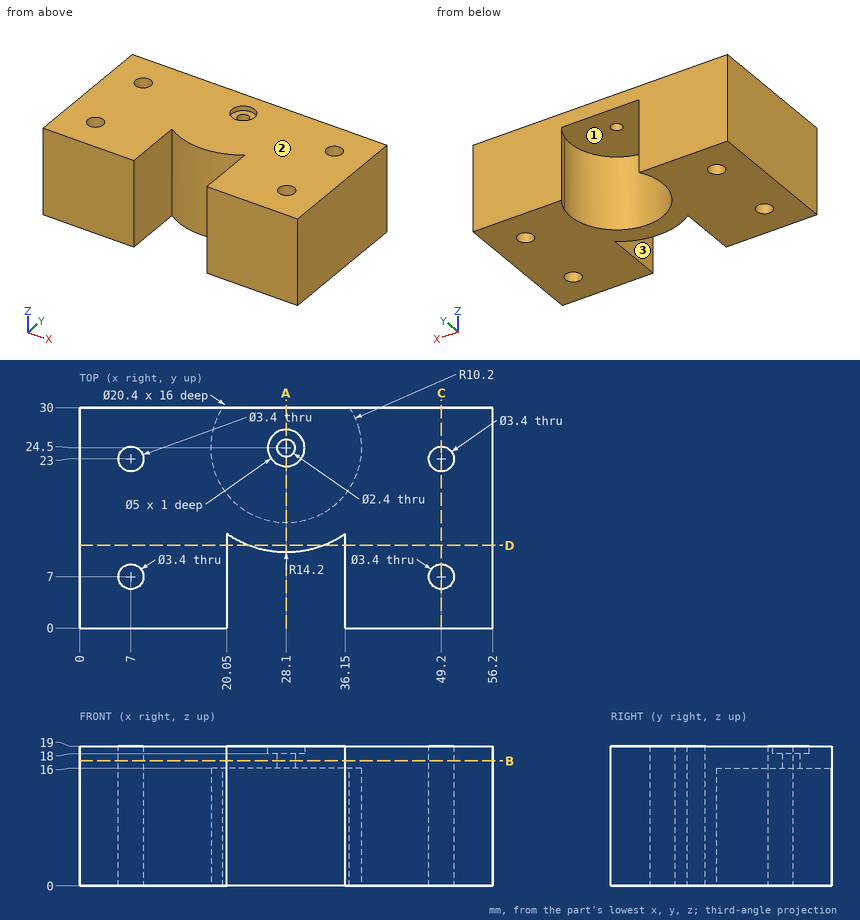
Print and shaded views of the part. All mm, measured from the part's lowest x, y and z. A direction names the side the tool comes from. Coordinates: 2 decimals unless noted, no trailing zeros. Write each loop counter-clockwise with the first axis right and the second up, starting at its lowest first coordinate (ties: lowest second). Pieces come first, ordered by that corner, then holes.
(1) Cut at B-B, the plane z = 17. List the corners of the cut face in (x, y), and give its area (3 significant figures).
(2) Flat gauge pins, fed straight in: pin 1 (5 mm diameter, centred on x = 33.5, z = 5.5, fed in from +Y); pin 2 (3 mm diameter, centred on x = 23, z = 9.5, fed in from +Y); pin 3 (12 mm diameter, centred on x = 28.1, y = 24.5, fed in from -Z). Where does each tip first touch, or does it go through?
(3) Drill centre lines: probe 1 along Y at (x, z) = (49.2, 7); probe 2 along Y at (x, z) = (28.1, 18.75); probe 3 along Y at (x, z) = (28.1, 17.5). Where is each one in solid material? Low to high.
(4) Cut at C-C, the plane x = 49.2. List the corners of the cut face in (y, z).
(5) 3-axis set-ups, long thin cutter, end or side, ignore diameter. For the marked faces 1, 2 and 3: which of +Z, -Z, +X, -X, +Y, -Y reach the whole face in a straight line?
(6) Cut at A-A, the plane x = 28.1. List the corners of the cut face in (y, z), and give its area (3 significant figures).
(7) Cut at D-D, the plane y = 11.25. List the corners of the cut face in (x, z).
Geometry says:
1. outline: (0, 0) - (20.05, 0) - (20.05, 12.8) arc R14.2 ccw to (36.15, 12.8) - (36.15, 0) - (56.2, 0) - (56.2, 30) - (0, 30) - close; hole circle Ø3.4 at (7, 7); hole circle Ø3.4 at (7, 23); hole circle Ø2.4 at (28.1, 24.5); hole circle Ø3.4 at (49.2, 7); hole circle Ø3.4 at (49.2, 23)
1. area: 1,470 mm2
2. pin 1: stops at y = 18.05
2. pin 2: stops at y = 16.72
2. pin 3: stops at z = 16
3. probe 1: y = 0 to 5.3, 8.7 to 21.3, 24.7 to 30
3. probe 2: y = 10.3 to 22, 27 to 30
3. probe 3: y = 10.3 to 23.3, 25.7 to 30
4. outline: (0, 0) - (5.3, 0) - (5.3, 19) - (0, 19) - close; (8.7, 0) - (21.3, 0) - (21.3, 19) - (8.7, 19) - close; (24.7, 0) - (30, 0) - (30, 19) - (24.7, 19) - close
5. face 1: -Z
5. face 2: +Z, +X, -X, +Y, -Y
5. face 3: +Z, -Z, -Y
6. outline: (10.3, 0) - (14.3, 0) - (14.3, 16) - (23.3, 16) - (23.3, 18) - (22, 18) - (22, 19) - (10.3, 19) - close; (25.7, 16) - (30, 16) - (30, 19) - (27, 19) - (27, 18) - (25.7, 18) - close
6. area: 113 mm2
7. outline: (0, 0) - (20.05, 0) - (20.05, 19) - (0, 19) - close; (22.99, 0) - (33.21, 0) - (33.21, 19) - (22.99, 19) - close; (36.15, 0) - (56.2, 0) - (56.2, 19) - (36.15, 19) - close
